```python
from build123d import *

# Parameters (mm, degrees)
SKETCH1_R                                       = 1.5
BOSS_EXTRUDE1_DEPTH                             = 4
CSK_FOR_M3_FLAT_HEAD_MACHINE_SCREW1_D           = 3.4
CSK_FOR_M3_FLAT_HEAD_MACHINE_SCREW1_DEPTH       = 7.5
CSK_FOR_M3_FLAT_HEAD_MACHINE_SCREW1_CSINK_D     = 6.3
CSK_FOR_M3_FLAT_HEAD_MACHINE_SCREW1_CSINK_ANGLE = 90
CSK_FOR_M3_FLAT_HEAD_MACHINE_SCREW1_TIP         = 1.021463052
FILLET1_R                                       = 2


with BuildPart() as part:
    # Sketch1 → Boss-Extrude1 (new body, symmetric)
    with BuildSketch(Plane(origin=(0, 0, 0), x_dir=(0, 0, -1), z_dir=(1, 0, 0))):
        with BuildLine():
            Line((0, -0.882843337), (0, 0))
            Line((0, 0), (0, 3.117156663))
            Line((0, 3.117156663), (-17.3820744, 3.117156663))
            Line((-17.3820744, 3.117156663), (-36.597884255, 47.117156663))
            Line((-36.597884255, 47.117156663), (-41, 47.117156663))
            ThreePointArc((-41, 47.117156663), (-45, 43.117156663), (-41, 39.117156663))
            Line((-41, 39.117156663), (-37.46891805, 39.117156663))
            Line((-37.46891805, 39.117156663), (-20, -0.882843337))
            Line((-20, -0.882843337), (0, -0.882843337))
        make_face()
        with Locations((-41, 43.117156663)):
            Circle(SKETCH1_R, mode=Mode.SUBTRACT)
    extrude(amount=BOSS_EXTRUDE1_DEPTH, both=True)

    # CSK for M3 Flat Head Machine Screw1
    with Locations(Plane(origin=(0, 3.117156663, 0), x_dir=(1, 0, 0), z_dir=(0, 1, 0))):
        with Locations((0, -13), (0, -4)):
            CounterSinkHole(CSK_FOR_M3_FLAT_HEAD_MACHINE_SCREW1_D / 2, CSK_FOR_M3_FLAT_HEAD_MACHINE_SCREW1_CSINK_D / 2, depth=CSK_FOR_M3_FLAT_HEAD_MACHINE_SCREW1_DEPTH, counter_sink_angle=CSK_FOR_M3_FLAT_HEAD_MACHINE_SCREW1_CSINK_ANGLE)
            with Locations((0, 0, -(CSK_FOR_M3_FLAT_HEAD_MACHINE_SCREW1_DEPTH + CSK_FOR_M3_FLAT_HEAD_MACHINE_SCREW1_TIP / 2))):  # 118° drill point
                Cone(0, CSK_FOR_M3_FLAT_HEAD_MACHINE_SCREW1_D / 2, CSK_FOR_M3_FLAT_HEAD_MACHINE_SCREW1_TIP, mode=Mode.SUBTRACT)

    # Fillet1
    fillet1_edges = [part.edges().sort_by_distance(p)[0] for p in [
        (0, 3.117156663, 17.3820744),
        (0, 39.117156663, 37.46891805),
    ]]
    fillet(fillet1_edges, radius=FILLET1_R)


solid = part.part
```
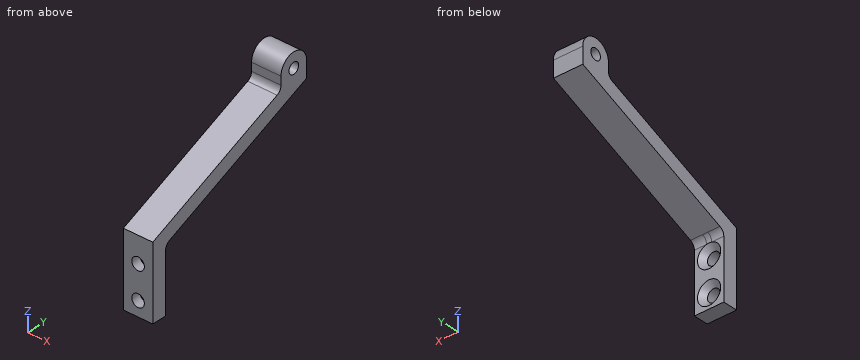
Check sheet for the modelled part. Datum: model origin and axes. Units: mm. Give positions to 0.01 mm unless a question says otherwise; leave off trailing zeros. Order: outer loops, then holes, each group sorted by start corner. A loop starts at its lowest first (then second) coordinate and runs counter-clockwise, first axis right, second up. Notation, with made-up numbers: M -36,86.5 L -2,86.5 A26 cw -2,121.5 Z; hole C 53,0.5 d8. An arc over 180 degrees is marked long. Answer in a Markdown table with one row per item.
1) Cross-section at D-D, the plane y = 16.5. Enter the section's corners in (x, z), plus the area to 3 significant figures.
Filled sheet:
| item | result |
|---|---|
| outline | M -4,23.23 L 4,23.23 L 4,27.59 L -4,27.59 Z |
| area | 34.9 mm2 |
2) Cross-section at A-A, the plane z = 4. Enter the section's corners in (x, y).
Filled sheet:
| item | result |
|---|---|
| outline | M -4,-0.88 L -1.7,-0.88 L -1.7,1.67 L -3.15,3.12 L -4,3.12 Z; M 1.7,-0.88 L 4,-0.88 L 4,3.12 L 3.15,3.12 L 1.7,1.67 Z |
3) Thickness scan on L1, parallel to Y at x = -0.75, z = 41; L2, parallel to X at y = 0.55, z = 13; L3, parallel to Z at x = 0, y = 0. Record the ranges inside material, lowest first. Write a range as [from, to].
Filled sheet:
| item | result |
|---|---|
| L1 | y = [39.12, 41.62], [44.62, 47.12] |
| L2 | x = [-4, -1.7], [1.7, 4] |
| L3 | z = [0, 2.3], [5.7, 11.3], [14.7, 20.39] |
4) Cross-section at B-B, the plane x = 0. Count the separate pieces of the cut face and the enclosed holes in it, plus the area to 3 significant figures.
Filled sheet:
| item | result |
|---|---|
| separate pieces | 3 |
| enclosed holes | 1 |
| area | 277 mm2 |
5) Gauge pin test, flat ends, axial feed: P1, Ø4, axis at x = 2, z = 11.5, coming from the +Y side; P2, Ø4, axis at x = -2, z = 24.5, coming from the -Y side; P3, Ø4, axis at x = 0, z = 13, coming from the +Y side. Record the tip position at first contact, or that the pin passes through.
Filled sheet:
| item | result |
|---|---|
| P1 | stops at y = 3.12 |
| P2 | stops at y = 4.84 |
| P3 | stops at y = 1.97 |
6) Cross-section at C-C, the plane z = 35. Enter the section's corners in (x, y), plus the area to 3 significant figures.
Filled sheet:
| item | result |
|---|---|
| outline | M -4,33.46 L 4,33.46 L 4,43.46 L -4,43.46 Z |
| area | 80.0 mm2 |
